Read the model definition and answer for the solid it produces. Units are mm, in the model's axes. A direction names the side the tool comes from. Round coordinates to 2 decimals unless told otherwise and drop trailing zeros. Loops run counter-clockwise (first coordinate to the right, second up) from the corner with the lowest first, then second, coordinate; pieces in that order, holes last. Notation, with made-up numbers: (28, 49.25) -> (66, 49.25) arc R8 cw to (66, 58.25) -> close; hole circle Ø3 at (14.25, 67.25). An arc over 180 degrees is marked (long way). Put each result on its own line as item: value.
from build123d import *

# Parameters (mm, degrees)
BOSS_EXTRUDE1_DEPTH = 20
FILLET1_R           = 3
SKETCH3_R           = 1.75
CUT_EXTRUDE1_DEPTH  = 24.600847442
SKETCH4_R           = 0.75
CUT_EXTRUDE2_DEPTH  = 24.430749028


with BuildPart() as part:
    # Sketch2 → Boss-Extrude1 (new body)
    with BuildSketch(Plane(origin=(0, 0, 0), x_dir=(1, 0, 0), z_dir=(0, 1, 0))):
        with BuildLine():
            Line((-1, 7), (1, 7))
            Line((1, 7), (1, 1.75))
            ThreePointArc((1, 1.75), (0.194543648, -0.194543648), (-1.75, -1))
            Line((-1.75, -1), (-11, -1))
            Line((-11, -1), (-11, 1))
            Line((-11, 1), (-1.75, 1))
            ThreePointArc((-1.75, 1), (-1.219669914, 1.219669914), (-1, 1.75))
            Line((-1, 1.75), (-1, 7))
        make_face()
    extrude(amount=BOSS_EXTRUDE1_DEPTH)

    # Fillet1
    fillet1_edges = [part.edges().sort_by_distance(p)[0] for p in [
        (-11, 0, 0),
        (-11, 20, 0),
        (0, 20, -7),
        (0, 0, -7),
    ]]
    fillet(fillet1_edges, radius=FILLET1_R)

    # Sketch3 → Cut-Extrude1 (cut, through all)
    with BuildSketch(Plane(origin=(0, 0, -1), x_dir=(-1, 0, 0), z_dir=(0, 0, -1))):
        with Locations((7, 16)):
            Circle(SKETCH3_R)
        with Locations((7, 4)):
            Circle(SKETCH3_R)
    extrude(amount=-CUT_EXTRUDE1_DEPTH, mode=Mode.SUBTRACT)

    # Sketch4 → Cut-Extrude2 (cut, through all)
    with BuildSketch(Plane.ZY.offset(1)):
        with Locations((-5, 10)):
            Circle(SKETCH4_R)
    extrude(amount=-CUT_EXTRUDE2_DEPTH, mode=Mode.SUBTRACT)


solid = part.part
Item 1: For a pull along Z with two mould halves and no side action, classify faces 1 (the cylindrical face through (0.01, 19.1, -6.14)), 2 (the cylindrical face through (-0.01, 10.51, -5.55)), 3 (the flat face through (-2, 0, 0)) as pulls with the +Z half, pulls with the -Z half, needs draft (parallel to the pull), parting line crosses it, or undercut.
Derived:
face 1: pulls with the -Z half
face 2: undercut
face 3: needs draft
Item 2: Find the intervals of material crossed by line 1 along Y through (x, z) = (-7, 0.45); line 2 along Y through (x, z) = (-7.75, -0.75); line 3 along Z through (x, y) = (-3.5, 15.75), in increasing order.
Derived:
line 1: y = 0 to 2.25, 5.75 to 14.25, 17.75 to 20
line 2: y = 0 to 2.42, 5.58 to 14.42, 17.58 to 20
line 3: z = -1 to 1
Item 3: Which of the six approach directions +Z, -Z, +X, -X, +Y, -Y give full straight-line access (tool end or side, diameter ignored) to faces 4 (the flat face through (-6, 10, -1)), 5 (the cylindrical face through (0.01, 0.9, -6.14))?
Derived:
face 4: -Z, -X, +Y, -Y
face 5: -Z, +X, -X, -Y
Item 4: The part is cut by section B-B (x = -7). Determine the outline of the cut face in (y, z).
Derived:
outline: (0, -1) -> (2.25, -1) -> (2.25, 1) -> (0, 1) -> close; (5.75, -1) -> (14.25, -1) -> (14.25, 1) -> (5.75, 1) -> close; (17.75, -1) -> (20, -1) -> (20, 1) -> (17.75, 1) -> close
Item 5: Flat-ended cylindrical pins translate along their axes: pin 1 Ø5.5 at (x, y) = (-7, 4) entering from -Z; pin 2 Ø1.4 at (y, z) = (10, -5) entering from -X; pin 3 Ø4 at (y, z) = (8, -3.5) entering from -X. Find the tip coordinate at first contact, or state that the pin passes through.
Derived:
pin 1: stops at z = -1
pin 2: passes through
pin 3: stops at x = -1.04
Item 6: The part is cut by section D-D (y = 4). Determine the outline of the cut face in (x, z), then the cut area to 3 significant figures.
Derived:
outline: (-11, -1) -> (-8.75, -1) -> (-8.75, 1) -> (-11, 1) -> close; (-5.25, -1) -> (-1.75, -1) arc R0.75 cw to (-1, -1.75) -> (-1, -7) -> (1, -7) -> (1, -1.75) arc R2.75 ccw to (-1.75, 1) -> (-5.25, 1) -> close
area: 27.5 mm^2
Item 7: The part is cut by section C-C (z = -5). Determine the outline of the cut face in (x, y), then the cut area to 3 significant figures.
Derived:
outline: (-1, 0.17) -> (1, 0.17) -> (1, 9.25) -> (-1, 9.25) -> close; (-1, 10.75) -> (1, 10.75) -> (1, 19.83) -> (-1, 19.83) -> close
area: 36.3 mm^2
Item 8: The part is cut by section A-A (y = 10). Determine the outline of the cut face in (x, z).
Derived:
outline: (-11, -1) -> (-1.75, -1) arc R0.75 cw to (-1, -1.75) -> (-1, -4.25) -> (1, -4.25) -> (1, -1.75) arc R2.75 ccw to (-1.75, 1) -> (-11, 1) -> close; (-1, -7) -> (1, -7) -> (1, -5.75) -> (-1, -5.75) -> close
